For this review, take the finished solid that the model builds, in its own axes (mm). Face numbers are marked on the shaded views. A direction names the side the tool comes from. Coordinates: 2 decimals unless noted, no trailing zeros. Loops run counter-clockwise (first coordinate to the right, second up) from the corner with the lowest first, then second, coordinate; pieces in that order, holes last. Notation, with made-up numbers: (16, -26) -> (58, -26) arc R36 cw to (58, 8) -> close; hole circle Ø9 at (-10.5, 8). An arc over 180 degrees is marked (long way). Answer in a Markdown table with one row per item.
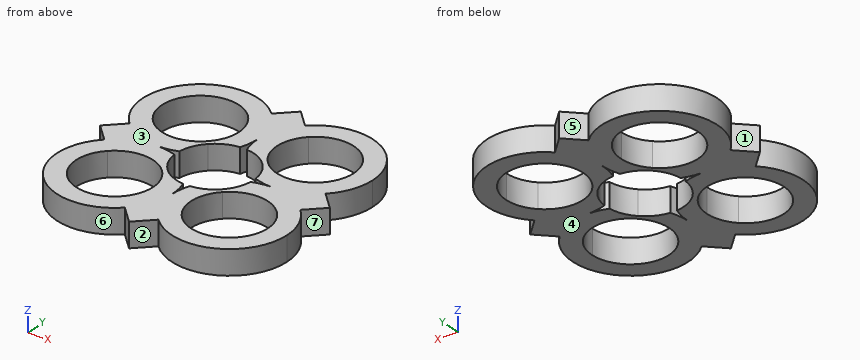
from build123d import *

# Parameters (mm, degrees)
F1_DEPTH = 7


with BuildPart() as f1:
    # F0 (on Top) → F1 (new body)
    with BuildSketch(Plane.XY):
        with BuildLine():
            ThreePointArc((7.7781745931, 7.7781745931), (9.9694294001, 4.6487070714), (10.9581597192, 0.9585069475))
            ThreePointArc((10.9581597192, 0.9585069475), (13.6879398448, 0.2413925048), (16.5, 0))
            ThreePointArc((16.5, 0), (22.814276634, 1.2559877136), (28.1672618896, 4.8327381104))
            Line((28.1672618896, 4.8327381104), (24.2781745931, 8.7218254069))
            ThreePointArc((24.2781745931, 8.7218254069), (16.5, 5.5), (8.7218254069, 8.7218254069))
            Line((8.7218254069, 8.7218254069), (7.7781745931, 7.7781745931))
        make_face()
        with BuildLine():
            ThreePointArc((16.5, 0), (13.6879398448, -0.2413925048), (10.9581597192, -0.9585069475))
            ThreePointArc((10.9581597192, -0.9585069475), (9.9694294001, -4.6487070714), (7.7781745931, -7.7781745931))
            Line((7.7781745931, -7.7781745931), (8.7218254069, -8.7218254069))
            ThreePointArc((8.7218254069, -8.7218254069), (16.5, -5.5), (24.2781745931, -8.7218254069))
            Line((24.2781745931, -8.7218254069), (28.1672618896, -4.8327381104))
            ThreePointArc((28.1672618896, -4.8327381104), (22.814276634, -1.2559877136), (16.5, 0))
        make_face()
        with BuildLine():
            ThreePointArc((28.1672618896, 4.8327381104), (22.814276634, 1.2559877136), (16.5, 0))
            Line((16.5, 0), (33, 0))
            Line((33, 0), (28.1672618896, 4.8327381104))
        make_face()
        with BuildLine():
            Line((33, 0), (16.5, 0))
            ThreePointArc((16.5, 0), (22.814276634, -1.2559877136), (28.1672618896, -4.8327381104))
            Line((28.1672618896, -4.8327381104), (33, 0))
        make_face()
        with BuildLine():
            ThreePointArc((0.9585069475, 10.9581597192), (4.6487070714, 9.9694294001), (7.7781745931, 7.7781745931))
            Line((7.7781745931, 7.7781745931), (8.7218254069, 8.7218254069))
            ThreePointArc((8.7218254069, 8.7218254069), (5.5, 16.5), (8.7218254069, 24.2781745931))
            Line((8.7218254069, 24.2781745931), (4.8327381104, 28.1672618896))
            ThreePointArc((4.8327381104, 28.1672618896), (1.2559877136, 22.814276634), (0, 16.5))
            ThreePointArc((0, 16.5), (0.2413925048, 13.6879398448), (0.9585069475, 10.9581597192))
        make_face()
        with BuildLine():
            Line((8.7218254069, -8.7218254069), (7.7781745931, -7.7781745931))
            ThreePointArc((7.7781745931, -7.7781745931), (4.6487070714, -9.9694294001), (0.9585069475, -10.9581597192))
            ThreePointArc((0.9585069475, -10.9581597192), (0.2413925048, -13.6879398448), (0, -16.5))
            ThreePointArc((0, -16.5), (1.2559877136, -22.814276634), (4.8327381104, -28.1672618896))
            Line((4.8327381104, -28.1672618896), (8.7218254069, -24.2781745931))
            ThreePointArc((8.7218254069, -24.2781745931), (5.5, -16.5), (8.7218254069, -8.7218254069))
        make_face()
        with BuildLine():
            Line((24.2781745931, 8.7218254069), (28.1672618896, 4.8327381104))
            ThreePointArc((28.1672618896, 4.8327381104), (31.7440122864, 10.185723366), (33, 16.5))
            ThreePointArc((33, 16.5), (31.7440122864, 22.814276634), (28.1672618896, 28.1672618896))
            Line((28.1672618896, 28.1672618896), (24.2781745931, 24.2781745931))
            ThreePointArc((24.2781745931, 24.2781745931), (26.6626748576, 20.709517756), (27.5, 16.5))
            ThreePointArc((27.5, 16.5), (26.6626748576, 12.290482244), (24.2781745931, 8.7218254069))
        make_face()
        with BuildLine():
            ThreePointArc((33, -16.5), (31.7440122864, -10.185723366), (28.1672618896, -4.8327381104))
            Line((28.1672618896, -4.8327381104), (24.2781745931, -8.7218254069))
            ThreePointArc((24.2781745931, -8.7218254069), (26.6626748576, -12.290482244), (27.5, -16.5))
            ThreePointArc((27.5, -16.5), (20.709517756, -26.6626748576), (8.7218254069, -24.2781745931))
            Line((8.7218254069, -24.2781745931), (4.8327381104, -28.1672618896))
            ThreePointArc((4.8327381104, -28.1672618896), (22.814276634, -31.7440122864), (33, -16.5))
        make_face()
        with BuildLine():
            Line((-8.7218254069, -8.7218254069), (-7.7781745931, -7.7781745931))
            ThreePointArc((-7.7781745931, -7.7781745931), (-9.9694294001, -4.6487070714), (-10.9581597192, -0.9585069475))
            ThreePointArc((-10.9581597192, -0.9585069475), (-13.6879398448, -0.2413925048), (-16.5, 0))
            ThreePointArc((-16.5, 0), (-22.814276634, -1.2559877136), (-28.1672618896, -4.8327381104))
            Line((-28.1672618896, -4.8327381104), (-24.2781745931, -8.7218254069))
            ThreePointArc((-24.2781745931, -8.7218254069), (-16.5, -5.5), (-8.7218254069, -8.7218254069))
        make_face()
        with BuildLine():
            ThreePointArc((-0.9585069475, -10.9581597192), (-4.6487070714, -9.9694294001), (-7.7781745931, -7.7781745931))
            Line((-7.7781745931, -7.7781745931), (-8.7218254069, -8.7218254069))
            ThreePointArc((-8.7218254069, -8.7218254069), (-6.3373251424, -12.290482244), (-5.5, -16.5))
            ThreePointArc((-5.5, -16.5), (-6.3373251424, -20.709517756), (-8.7218254069, -24.2781745931))
            Line((-8.7218254069, -24.2781745931), (-4.8327381104, -28.1672618896))
            ThreePointArc((-4.8327381104, -28.1672618896), (-1.2559877136, -22.814276634), (0, -16.5))
            ThreePointArc((0, -16.5), (-0.2413925048, -13.6879398448), (-0.9585069475, -10.9581597192))
        make_face()
        with BuildLine():
            ThreePointArc((-16.5, 0), (-13.6879398448, 0.2413925048), (-10.9581597192, 0.9585069475))
            ThreePointArc((-10.9581597192, 0.9585069475), (-9.9694294001, 4.6487070714), (-7.7781745931, 7.7781745931))
            Line((-7.7781745931, 7.7781745931), (-8.7218254069, 8.7218254069))
            ThreePointArc((-8.7218254069, 8.7218254069), (-16.5, 5.5), (-24.2781745931, 8.7218254069))
            Line((-24.2781745931, 8.7218254069), (-28.1672618896, 4.8327381104))
            ThreePointArc((-28.1672618896, 4.8327381104), (-22.814276634, 1.2559877136), (-16.5, 0))
        make_face()
        with BuildLine():
            ThreePointArc((-28.1672618896, -4.8327381104), (-22.814276634, -1.2559877136), (-16.5, 0))
            Line((-16.5, 0), (-33, 0))
            Line((-33, 0), (-28.1672618896, -4.8327381104))
        make_face()
        with BuildLine():
            Line((-33, 0), (-16.5, 0))
            ThreePointArc((-16.5, 0), (-22.814276634, 1.2559877136), (-28.1672618896, 4.8327381104))
            Line((-28.1672618896, 4.8327381104), (-33, 0))
        make_face()
        with BuildLine():
            ThreePointArc((-7.7781745931, 7.7781745931), (-4.6487070714, 9.9694294001), (-0.9585069475, 10.9581597192))
            ThreePointArc((-0.9585069475, 10.9581597192), (-0.2413925048, 13.6879398448), (0, 16.5))
            ThreePointArc((0, 16.5), (-1.2559877136, 22.814276634), (-4.8327381104, 28.1672618896))
            Line((-4.8327381104, 28.1672618896), (-8.7218254069, 24.2781745931))
            ThreePointArc((-8.7218254069, 24.2781745931), (-6.3373251424, 20.709517756), (-5.5, 16.5))
            ThreePointArc((-5.5, 16.5), (-6.3373251424, 12.290482244), (-8.7218254069, 8.7218254069))
            Line((-8.7218254069, 8.7218254069), (-7.7781745931, 7.7781745931))
        make_face()
        with BuildLine():
            ThreePointArc((-4.8327381104, 28.1672618896), (-1.2559877136, 22.814276634), (0, 16.5))
            ThreePointArc((0, 16.5), (1.2559877136, 22.814276634), (4.8327381104, 28.1672618896))
            Line((4.8327381104, 28.1672618896), (0, 33))
            Line((0, 33), (-4.8327381104, 28.1672618896))
        make_face()
        with BuildLine():
            Line((4.8327381104, 28.1672618896), (8.7218254069, 24.2781745931))
            ThreePointArc((8.7218254069, 24.2781745931), (16.5, 27.5), (24.2781745931, 24.2781745931))
            Line((24.2781745931, 24.2781745931), (28.1672618896, 28.1672618896))
            ThreePointArc((28.1672618896, 28.1672618896), (16.5, 33), (4.8327381104, 28.1672618896))
        make_face()
        with BuildLine():
            ThreePointArc((4.8327381104, -28.1672618896), (1.2559877136, -22.814276634), (0, -16.5))
            ThreePointArc((0, -16.5), (-1.2559877136, -22.814276634), (-4.8327381104, -28.1672618896))
            Line((-4.8327381104, -28.1672618896), (0, -33))
            Line((0, -33), (4.8327381104, -28.1672618896))
        make_face()
        with BuildLine():
            ThreePointArc((-4.8327381104, 28.1672618896), (-28.1672618896, 28.1672618896), (-28.1672618896, 4.8327381104))
            Line((-28.1672618896, 4.8327381104), (-24.2781745931, 8.7218254069))
            ThreePointArc((-24.2781745931, 8.7218254069), (-24.2781745931, 24.2781745931), (-8.7218254069, 24.2781745931))
            Line((-8.7218254069, 24.2781745931), (-4.8327381104, 28.1672618896))
        make_face()
        with BuildLine():
            Line((-24.2781745931, -8.7218254069), (-28.1672618896, -4.8327381104))
            ThreePointArc((-28.1672618896, -4.8327381104), (-28.1672618896, -28.1672618896), (-4.8327381104, -28.1672618896))
            Line((-4.8327381104, -28.1672618896), (-8.7218254069, -24.2781745931))
            ThreePointArc((-8.7218254069, -24.2781745931), (-24.2781745931, -24.2781745931), (-24.2781745931, -8.7218254069))
        make_face()
    extrude(amount=F1_DEPTH)


solid = f1.part
Item 1: Take a section at B-B, the plane y = 2. State the section outline as (x, z) points.
Worked answers:
| item | result |
|---|---|
| outline | (-31, 0) -> (-10.82, 0) -> (-10.82, 7) -> (-31, 7) -> close; (10.82, 0) -> (31, 0) -> (31, 7) -> (10.82, 7) -> close |
Item 2: Take a section at D-D, the plane y = 18. State the section outline as (x, z) points.
Worked answers:
| item | result |
|---|---|
| outline | (-32.93, 0) -> (-27.4, 0) -> (-27.4, 7) -> (-32.93, 7) -> close; (-5.6, 0) -> (5.6, 0) -> (5.6, 7) -> (-5.6, 7) -> close; (27.4, 0) -> (32.93, 0) -> (32.93, 7) -> (27.4, 7) -> close |
Item 3: Insertion check: pin 1 (1.5 mm diameter, centred on x = -11.5, z = 5.5, fed in from +Y). The pin has a flat end and moves straight along its axis. Give the tip position at first contact, or say it passes through.
Worked answers:
| item | result |
|---|---|
| pin 1 | y = 32.44 |
Item 4: Take a section at C-C, the plane x = 21.5. State the section outline as (y, z) points, and give its area (3 significant figures).
Worked answers:
| item | result |
|---|---|
| outline | (-32.22, 0) -> (-26.3, 0) -> (-26.3, 7) -> (-32.22, 7) -> close; (-6.7, 0) -> (6.7, 0) -> (6.7, 7) -> (-6.7, 7) -> close; (26.3, 0) -> (32.22, 0) -> (32.22, 7) -> (26.3, 7) -> close |
| area | 177 mm² |
Item 5: Take a section at A-A, the plane x = -4. State the section outline as (y, z) points, and give its area (3 significant figures).
Worked answers:
| item | result |
|---|---|
| outline | (-29, 0) -> (-10.25, 0) -> (-10.25, 7) -> (-29, 7) -> close; (10.25, 0) -> (29, 0) -> (29, 7) -> (10.25, 7) -> close |
| area | 263 mm² |
Item 6: For L1, parallel to Y at x = 17, z = 0.5; L2, parallel to X at y = -25.5, z = 3.5; L3, parallel to Y at x = -18, z = 6, list the stretches that pass through material, from the lowest coordinate up.
Worked answers:
| item | result |
|---|---|
| L1 | -32.99 to -27.49, -5.51 to 5.51, 27.49 to 32.99 |
| L2 | -30.33 to -22.82, -10.18 to 10.18, 22.82 to 30.33 |
| L3 | -32.93 to -27.4, -5.6 to 5.6, 27.4 to 32.93 |
Item 7: For the marked faces 1, 2 and 3, list the 3-axis set-ups (+Z, -Z, +X, -X, +Y, -Y) from which the entire face can be reached by the end or side of a thin tool; tool diameter is ignored.
Worked answers:
| item | result |
|---|---|
| face 1 | +Z, -Z, -X |
| face 2 | +Z, -Z, -Y |
| face 3 | +Z, +X, -X, +Y, -Y |
Item 8: The part is to be moulded in two halves that separate along X. For the marked faces 4, 5, 6 and 7, say which applies: +X half, -X half, draft (parallel to the pull), parting line (faces both ways), or undercut.
Worked answers:
| item | result |
|---|---|
| face 4 | draft |
| face 5 | undercut |
| face 6 | undercut |
| face 7 | +X half |
